Read the model definition and answer for the solid it produces. Units are mm, in the model's axes. Face numbers are marked on the shaded views. A direction names the side the tool comes from. Coordinates: 2 decimals unless noted, no trailing zeros. Write each loop counter-clockwise with the first axis right and the second up, starting at its lowest first coordinate (ties: lowest second). Pieces come first, ordered by that corner, then holes. Notation, with made-up numbers: (-31.5, 63.25) -> (-3.5, 63.25) arc R28 ccw to (-3.5, 97.25) -> close; hole circle Ø2 at (82.5, 3). An arc over 180 degrees is marked (long way). Use CSV: the item, a comma, the result in double quotes.
from build123d import *

# Parameters (mm, degrees)
SKETCH_1_W                = 40
SKETCH_1_H                = 48
SKETCH_1_R                = 1.75
EXTRUDE_1_DEPTH           = 4
SKETCH_2_W                = 40
SKETCH_2_H                = 7.75
EXTRUDE_5_DEPTH           = 20.5
SKETCH_4_W                = 40
SKETCH_4_H                = 36
EXTRUDE_6_DEPTH           = 3
FILLET_4_R                = 5
FILLET_5_R                = 5
FILLET_7_R                = 2
FILLET_8_R                = 2
CUT_EXTRUDE_START         = -27.5
CUT_EXTRUDE_1_OUTLINE_R   = 1.75
CUT_EXTRUDE_1_OUTLINE_R_2 = 2.15
CUT_EXTRUDE_1_DEPTH       = 27.5
FILLET_9_R                = 1
FILLET_10_R               = 1
SKETCH_6_R                = 2.45
CUT_EXTRUDE_2_DEPTH       = 42.620307543


# Read off the part's stored shape, not the designer's step: 切除-拉伸1
with BuildPart() as part:
    # 草图1 → 凸台-拉伸1 (new body)
    with BuildSketch(Plane(origin=(0, 0, 0), x_dir=(1, 0, 0), z_dir=(0, 1, 0))):
        Rectangle(SKETCH_1_W, SKETCH_1_H)
        with Locations(Location((11.45, 14, 0), (0, 0, 270))):
            Circle(SKETCH_1_R, mode=Mode.SUBTRACT)
        with Locations(Location((-11.45, 14, 0), (0, 0, 270))):
            Circle(SKETCH_1_R, mode=Mode.SUBTRACT)
        with Locations(Location((-11.45, -14, 0), (0, 0, 270))):
            Circle(SKETCH_1_R, mode=Mode.SUBTRACT)
        with Locations(Location((11.45, -14, 0), (0, 0, 270))):
            Circle(SKETCH_1_R, mode=Mode.SUBTRACT)
        with BuildLine():
            Line((-2.45, -15.5), (-2.45, 15.5))
            ThreePointArc((-2.45, 15.5), (0, 17.95), (2.45, 15.5))
            Line((2.45, 15.5), (2.45, -15.5))
            ThreePointArc((2.45, -15.5), (0, -17.95), (-2.45, -15.5))
        make_face(mode=Mode.SUBTRACT)
    extrude(amount=EXTRUDE_1_DEPTH)

    # 草图2 → 凸台-拉伸5 (add)
    with BuildSketch(Plane(origin=(0, 4, 0), x_dir=(1, 0, 0), z_dir=(0, 1, 0))):
        with Locations((0, -14.125)):
            Rectangle(SKETCH_2_W, SKETCH_2_H)
        with Locations((0, 14.125)):
            Rectangle(SKETCH_2_W, SKETCH_2_H)
    extrude(amount=EXTRUDE_5_DEPTH)

    # 草图4 → 凸台-拉伸6 (add)
    with BuildSketch(Plane(origin=(0, 24.5, 0), x_dir=(1, 0, 0), z_dir=(0, 1, 0))):
        Rectangle(SKETCH_4_W, SKETCH_4_H)
    extrude(amount=EXTRUDE_6_DEPTH)

    # 圆角4
    fillet_4_edges = [part.edges().sort_by_distance(p)[0] for p in [
        (0, 4, -18),
    ]]
    fillet(fillet_4_edges, radius=FILLET_4_R)

    # 圆角5
    fillet_5_edges = [part.edges().sort_by_distance(p)[0] for p in [
        (0, 4, 18),
    ]]
    fillet(fillet_5_edges, radius=FILLET_5_R)

    # 圆角7
    fillet_7_edges = [part.edges().sort_by_distance(p)[0] for p in [
        (0, 0, 24),
    ]]
    fillet(fillet_7_edges, radius=FILLET_7_R)

    # 圆角8
    fillet_8_edges = [part.edges().sort_by_distance(p)[0] for p in [
        (0, 0, -24),
    ]]
    fillet(fillet_8_edges, radius=FILLET_8_R)

    # 切除-拉伸1 outline → 切除-拉伸1 (cut)
    with BuildSketch(Plane.XZ.offset(CUT_EXTRUDE_START)):
        with Locations((-11.45, 14)):
            Circle(CUT_EXTRUDE_1_OUTLINE_R)
        with Locations((-11.45, -14)):
            Circle(CUT_EXTRUDE_1_OUTLINE_R)
        with Locations((11.45, -14)):
            Circle(CUT_EXTRUDE_1_OUTLINE_R)
        with Locations((11.45, 14)):
            Circle(CUT_EXTRUDE_1_OUTLINE_R)
        with Locations((-11.45, 0)):
            Circle(CUT_EXTRUDE_1_OUTLINE_R_2)
        with Locations((11.45, 0)):
            Circle(CUT_EXTRUDE_1_OUTLINE_R_2)
    extrude(amount=CUT_EXTRUDE_1_DEPTH, mode=Mode.SUBTRACT)

    # 圆角9
    fillet_9_edges = [part.edges().sort_by_distance(p)[0] for p in [
        (0, 27.5, 18),
    ]]
    fillet(fillet_9_edges, radius=FILLET_9_R)

    # 圆角10
    fillet_10_edges = [part.edges().sort_by_distance(p)[0] for p in [
        (0, 27.5, -18),
    ]]
    fillet(fillet_10_edges, radius=FILLET_10_R)

    # 草图6 → 切除-拉伸2 (cut, through all)
    with BuildSketch(Plane.XZ):
        with Locations(Location((0, 0, 0), (0, 0, 270))):
            Circle(SKETCH_6_R)
    extrude(amount=-CUT_EXTRUDE_2_DEPTH, mode=Mode.SUBTRACT)


solid = part.part
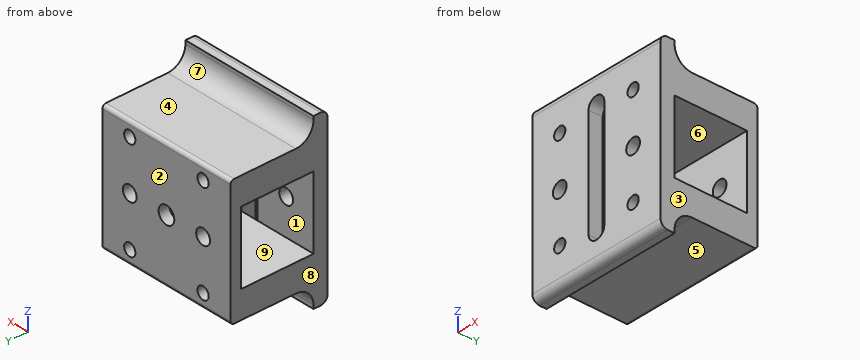
1. A cutting plane is placed at A-A (y = 11). Give the vertices of the cut face in (x, z).
Solutions:
outline,"(-20, -18) -> (20, -18) -> (20, -10.25) -> (-20, -10.25) -> close; (-20, 10.25) -> (20, 10.25) -> (20, 18) -> (-20, 18) -> close; hole circle Ø3.5 at (-11.45, -14); hole circle Ø3.5 at (-11.45, 14); hole circle Ø3.5 at (11.45, -14); hole circle Ø3.5 at (11.45, 14)"
2. A cutting plane is placed at B-B (z = 0). Give the number of separate pieces and of enclosed holes in the cut face, and give its area (4 significant figures).
Solutions:
separate pieces,"8"
enclosed holes,"0"
area,"185.5 mm^2"
3. Each of these flat-tipped pins is pushed along its axis until it touches: pin 1 Ø6 at (x, y) = (-7.5, 10) entering from +Z; pin 2 Ø5 at (x, y) = (-9, 18.5) entering from +Z; pin 3 Ø3 at (x, z) = (0, 0) entering from +Y; pin 4 Ø0.8 at (x, z) = (-1, 23.5) entering from +Y. Where does it stop, or does it pass through?
Solutions:
pin 1,"stops at z = 18.42"
pin 2,"stops at z = 18"
pin 3,"passes through"
pin 4,"stops at y = 4"
4. Find the intervals of material crossed by line 1 along Z through (x, y) = (-11.45, 26.8); line 2 along Z through (x, y) = (-11.45, 2); line 3 along X through (y, z) = (6.5, -14), in increasing order.
Solutions:
line 1,"z = -17.95 to -15.75, -12.25 to -2.15, 2.15 to 12.25, 15.75 to 17.95"
line 2,"z = -24 to -15.75, -12.25 to -2.15, 2.15 to 12.25, 15.75 to 24"
line 3,"x = -20 to -13.2, -9.7 to 9.7, 13.2 to 20"
5. For a pull along Z with two mould halves and no side action, classify the marked faces 6, 7, 8 and 9 as pulls with the +Z half, pulls with the -Z half, needs draft (parallel to the pull), parting line crosses it, or undercut.
Solutions:
face 6,"undercut"
face 7,"pulls with the +Z half"
face 8,"needs draft"
face 9,"undercut"
6. A cutting plane is placed at D-D (z = -8). Give the vertices of the cut face in (x, y).
Solutions:
outline,"(-20, 0) -> (-2.45, 0) -> (-2.45, 4) -> (-20, 4) -> close; (-20, 24.5) -> (20, 24.5) -> (20, 27.5) -> (-20, 27.5) -> close; (2.45, 0) -> (20, 0) -> (20, 4) -> (2.45, 4) -> close"
7. A tool of negligible diameter and unlimited length cuts with its end or side. For the marked faces 1, 2, 3, 4 and 5, from which of +Z, -Z, +X, -X, +Y, -Y can it reach the whole face along a straight path? Write none if from no direction.
Solutions:
face 1,"+X, -X"
face 2,"+Z, -Z, +X, -X, +Y"
face 3,"+Z, -Z, +X, +Y, -Y"
face 4,"+Z, +X, -X, +Y"
face 5,"-Z, +X, -X, +Y"
